The listing builds one solid part. Answer for the finished solid, in the listing's coordinates (mm). Face numbers are marked on the shaded views. A direction names the side the tool comes from. Give positions to 0.01 mm unless a question says otherwise; leave off trailing zeros. Loops run counter-clockwise (first coordinate to the right, second up) from the corner with the lowest first, then second, coordinate; pieces in that order, holes last. Notation, with made-up numbers: (46, -20) - (79, -20) arc R16 cw to (79, -8) - close; hole circle Ø5 at (3.5, 67). An arc over 180 degrees is marked (long way). Write each question's results on one line, items separated by ' | '.
from build123d import *

# Parameters (mm, degrees)
SKETCH1_W                = 25.4
SKETCH1_H                = 12.7
BOSS_EXTRUDE1_DEPTH      = 1.27
FILLET1_R                = 0.2286
BOSS_EXTRUDE2_DEPTH      = 15.24
BOSS_EXTRUDE2_DEPTH_BACK = 15.24


with BuildPart() as part:
    # Sketch1 → Boss-Extrude1 (new, symmetric)
    with BuildSketch(Plane(origin=(0, 0, 0), x_dir=(1, 0, 0), z_dir=(0, 1, 0))):
        Rectangle(SKETCH1_W, SKETCH1_H)
    extrude(amount=BOSS_EXTRUDE1_DEPTH, both=True)

    # Fillet1
    fillet1_edges = [part.edges().sort_by_distance(p)[0] for p in [
        (0, 1.27, 6.35),
        (0, -1.27, 6.35),
        (0, -1.27, -6.35),
        (0, 1.27, -6.35),
    ]]
    fillet(fillet1_edges, radius=FILLET1_R)

    # Sketch3 → Boss-Extrude2 (add, two sides: drawn at the far end of the back side and taken through both)
    with BuildSketch(Plane(origin=(0, 0, 0), x_dir=(0, 0, -1), z_dir=(1, 0, 0)).offset(-BOSS_EXTRUDE2_DEPTH_BACK)):
        with BuildLine():
            Line((-2.75846638, 0.890155409), (2.75846638, 0.890155409))
            ThreePointArc((2.75846638, 0.890155409), (3.648621789, 0), (2.75846638, -0.890155409))
            Line((2.75846638, -0.890155409), (-2.75846638, -0.890155409))
            ThreePointArc((-2.75846638, -0.890155409), (-3.648621789, 0), (-2.75846638, 0.890155409))
        make_face()
    extrude(amount=BOSS_EXTRUDE2_DEPTH + BOSS_EXTRUDE2_DEPTH_BACK)


solid = part.part
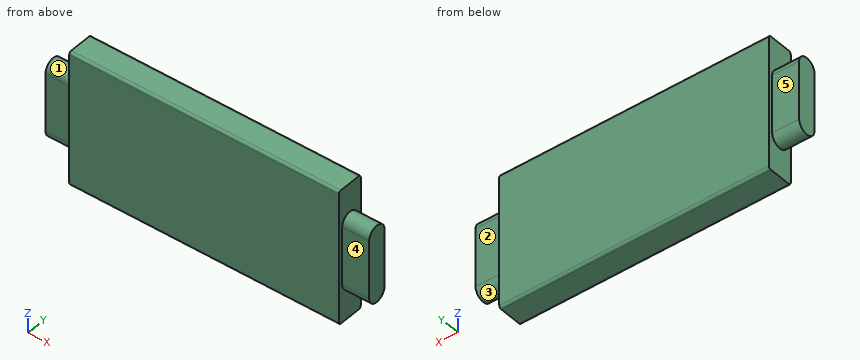
Item 1: Find the intervals of material crossed by line 1 along X through (y, z) = (-0.45, 5), in increasing order. Write a range as [from, to].
Values found:
line 1: x = [-12.7, 12.7]
Item 2: A cutting plane is placed at A-A, the plane y = 0. Determine the outline of the cut face in (x, z), plus the area to 3 significant figures.
Values found:
outline: (-15.24, -3.65) - (-12.7, -3.65) - (-12.7, -6.35) - (12.7, -6.35) - (12.7, -3.65) - (15.24, -3.65) - (15.24, 3.65) - (12.7, 3.65) - (12.7, 6.35) - (-12.7, 6.35) - (-12.7, 3.65) - (-15.24, 3.65) - close | area: 360 mm²
Item 3: For the marked faces 1, 2, 3, 4 and 5, determine the directions among +Z, -Z, +X, -X, +Y, -Y from which every point of the face is accessible in a straight line to the end or side of a thin tool.
Values found:
face 1: +Z, -X | face 2: +Z, -Z, +X, +Y | face 3: -Z, +X | face 4: +Z, -Z, +X, -Y | face 5: +Z, -Z, -X, +Y
Item 4: A cutting plane is placed at B-B, the plane z = 2. Determine the outline of the cut face in (x, y).
Values found:
outline: (-15.24, -0.89) - (-12.7, -0.89) - (-12.7, -1.27) - (12.7, -1.27) - (12.7, -0.89) - (15.24, -0.89) - (15.24, 0.89) - (12.7, 0.89) - (12.7, 1.27) - (-12.7, 1.27) - (-12.7, 0.89) - (-15.24, 0.89) - close
Item 5: A cutting plane is placed at C-C, the plane z = -4.5. Determine the outline of the cut face in (x, y), plus the area to 3 significant figures.
Values found:
outline: (-12.7, -1.27) - (12.7, -1.27) - (12.7, 1.27) - (-12.7, 1.27) - close | area: 64.5 mm²
Item 6: A flat-ended cylindrical pin translates along its axis: P1, Ø0.8, axis at x = 14, z = -1.5, coming from the +Y side. Find the tip coordinate at first contact, or state that the pin passes through.
Values found:
P1: stops at y = 0.89
